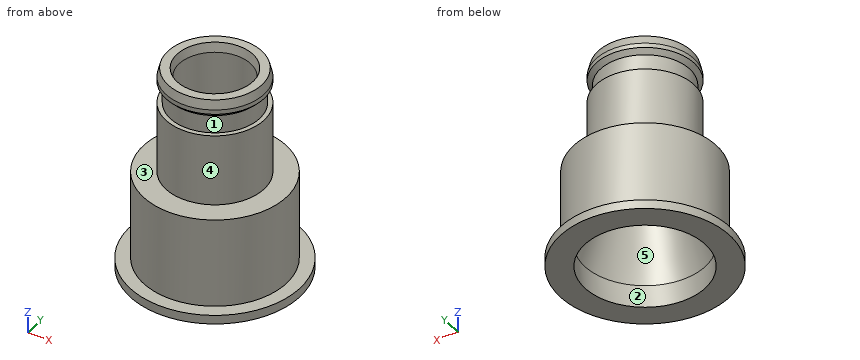
Autodesk Fusion 360 part; units mm, degrees
sketch "Skizze1" plane through (0, 0, 0) normal (1, 0, 0) x (0, 1, 0) in component "Schlauchadapter-22mm-40mm NATO"
  line L0 (0, -8) -> (0, 92) construction
  line L1 (0, 0) -> (19, 0) construction
  line L2 (13.5, -8.8503) -> (13.5, 10.0011) construction
  line L3 (16, -9) -> (16, -8)
  line L4 (16, -8) -> (16, 12.6517) construction
  line L5 (8, 9.6655) -> (8, 11)
  line L6 (8, 11) -> (8, 32.4994) construction
  line L7 (13.5, 0) -> (19, 0)
  line L8 (19, 0) -> (19, 2)
  line L9 (19, 2) -> (16, 2)
  line L10 (16, 2) -> (16, 22)
  line L11 (13.5, 0) -> (13.5, 5)
  line L12 (16, 22) -> (-10.2408, 22) construction
  line L13 (11, 9.9222) -> (11, 30.0778) construction
  line L14 (16, 22) -> (11, 22)
  line L15 (11, 22) -> (11, 38)
  line L16 (8, 28.4613) -> (8, 38.3723) construction
  line L17 (10, 31.378) -> (10, 40.0422) construction
  line L18 (11, 38) -> (10, 38)
  line L19 (10, 38) -> (10, 42)
  line L20 (11, 38) -> (-2.5, 38) construction
  line L21 (8, 22) -> (8, 38)
  line L22 (11, 22) -> (11, 43) construction
  line L23 (10, 42) -> (11, 42)
  line L24 (11, 42) -> (11, 46)
  line L25 (11, 46) -> (8, 46)
  line L26 (8, 46) -> (8, 38)
  line L27 (8, 22) -> (13.5, 5)
  dimension "d16" = 19
  dimension "d17" = 13.5
  dimension "d18" = 16
  dimension "d19" = 8
  dimension "d20" = 2
  dimension "d21" = 20
  dimension "d22" = 5
  dimension "d23" = 11
  dimension "d24" = 16
  dimension "d25" = 8
  dimension "d26" = 10
  dimension "d27" = 4
  dimension "d28" = 4
revolve "Drehen1" add sketch "Skizze1" angle 360 about axis through (0, 0, -8) along (0, 0, 1) in component "Schlauchadapter-22mm-40mm NATO"
chamfer "Fase1" distance 2 distance2 0.5 1 edges at (-10.2556, 3.9778, 46) measured on face at (0.5483, 10.9863, 43.3333) in component "Schlauchadapter-22mm-40mm NATO"
chamfer "Fase2" distance 1 angle 45 1 edges at (-10.2556, 3.9778, 42) in component "Schlauchadapter-22mm-40mm NATO"
chamfer "Fase4" distance 0.5 distance2 2 1 edges at (-7.4586, 2.8929, 46) measured on face at (0.9191, 9.5978, 46) in component "Schlauchadapter-22mm-40mm NATO"
component "Schlauchadapter-22mm-40mm NATO" placed x (1, 0, 0) y (0, 1, 0) z (0, 0, 1) at (0, 0, 0)
Geometry: final body of the model. Coordinates: model frame, mm. Face numbers are marked on the shaded views. A direction names the side the tool comes from. Give positions to 0.01 mm unless a question says otherwise; leave off trailing zeros. Order: outer loops, then holes, each group sorted by start corner. A loop starts at its lowest first (then second) coordinate and runs counter-clockwise, first axis right, second up. Notation, with made-up numbers: (56, 60.5) -> (95, 60.5) arc R13 cw to (95, 67.5) -> close; hole circle Ø5 at (58, 24.5). An arc over 180 degrees is marked (long way). Put each result on its own line as item: value.
Q1. Reachability of the marked faces 4 and 5 from +Z, -Z, +X, -X, +Y, -Y: full face, straight path, thin tool, end or side. Return the list, or none.
Here are the results:
face 4: +Z
face 5: -Z
Q2. Pin query (flat end, axial travel): pin 1 (10 mm diameter, centred on y = 2, z = 23, fed in from -X); pin 2 (4 mm diameter, centred on x = 6.5, z = 27, fed in from -Y); pin 3 (6 mm diameter, centred on y = 8, z = 20, fed in from +X). Return the tip coordinate at first contact, or that it passes through.
Here are the results:
pin 1: stops at x = -16
pin 2: stops at y = -10.04
pin 3: stops at x = 15.2
Q3. Draft query along X for the marked faces 1, 2 and 3. Return one class per face: released by +X, released by -X, zero draft, split by the parting line, or undercut.
Here are the results:
face 1: split by the parting line
face 2: undercut
face 3: zero draft
Q4. Material intervals for L1, parallel to Y at x = 0, z = 2.05; L2, parallel to Y at x = 0, z = 1.2; L3, parallel to X at y = 0, z = 32.5, sorted ascending.
Here are the results:
L1: y = -16 to -13.5, 13.5 to 16
L2: y = -19 to -13.5, 13.5 to 19
L3: x = -11 to -8, 8 to 11
Q5. Section C-C, the plane z = 23.5. Return loops of the section in (x, y), then the cut area to 3 significant figures.
Here are the results:
outline: circle Ø22 at (0, 0); hole circle Ø16 at (0, 0)
area: 179 mm^2
Q6. Section D-D, the plane z = 17.5. Return loops of the section in (x, y), then the cut area to 3 significant figures.
Here are the results:
outline: circle Ø32 at (0, 0); hole circle Ø18.91 at (0, 0)
area: 523 mm^2
